Input: part model. Units: mm. Frame: model coordinates. Face numbers are marked on the shaded views. A direction names the side the tool comes from. Coordinates: 2 decimals unless noted, no trailing zeros. Order: outer loops, then holes, each group sorted by start corner. A loop starts at its lowest first (then second) coordinate and runs counter-clockwise, first axis right, second up. Notation, with made-up numbers: (82, 50.25) -> (108, 50.25) arc R35 ccw to (108, 86.25) -> close; hole circle Ø6 at (-16, 53.25). An arc over 180 degrees is marked (long way). One line per question, with ' | ' between items.
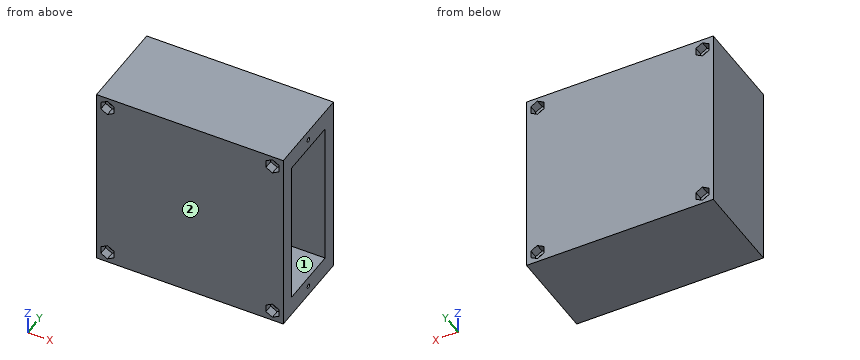
```python
from build123d import *

# Parameters (mm, degrees)
ESBO_O1_W                = 86
ESBO_O1_H                = 86
RESSALTO_EXTRUS_O1_DEPTH = 21
ESBO_O2_W                = 68
ESBO_O2_H                = 28
CORTE_EXTRUS_O1_DEPTH    = 78
ESBO_O6_R                = 1.65
CORTE_EXTRUS_O3_DEPTH    = 9
CORTE_EXTRUS_O4_DEPTH    = 4
ESPELHAR2_COPY_1_DEPTH   = 4
CORTE_EXTRUS_O5_START    = -9
ESBO_O8_R                = 1.65
CORTE_EXTRUS_O5_DEPTH    = 9
ESPELHAR4_COPY_1_DEPTH   = 4
ESPELHAR4_COPY_2_DEPTH   = 4
ESPELHAR4_COPY_3_DEPTH   = 4
ESBO_O9_R                = 1
CORTE_EXTRUS_O6_DEPTH    = 6


with BuildPart() as part:
    # Esboço1 → Ressalto-extrusão1 (new, symmetric)
    with BuildSketch(Plane(origin=(0, 0, 0), x_dir=(1, 0, 0), z_dir=(0, 1, 0))):
        Rectangle(ESBO_O1_W, ESBO_O1_H)
    extrude(amount=RESSALTO_EXTRUS_O1_DEPTH, both=True)

    # Esboço2 → Corte-extrusão1 (cut)
    with BuildSketch(Plane(origin=(43, 0, 0), x_dir=(0, 0, -1), z_dir=(1, 0, 0))):
        Rectangle(ESBO_O2_W, ESBO_O2_H)
    extrude(amount=-CORTE_EXTRUS_O1_DEPTH, mode=Mode.SUBTRACT)

    # Esboço6 → Corte-extrusão3 (cut)
    with BuildSketch(Plane(origin=(0, 21, 0), x_dir=(1, 0, 0), z_dir=(0, 1, 0))):
        with Locations(Location((-38, -38, 0), (0, 0, 270))):
            Circle(ESBO_O6_R)
        with Locations(Location((-38, 38, 0), (0, 0, 270))):
            Circle(ESBO_O6_R)
        with Locations(Location((38, 38, 0), (0, 0, 270))):
            Circle(ESBO_O6_R)
        with Locations(Location((38, -38, 0), (0, 0, 270))):
            Circle(ESBO_O6_R)
    extrude(amount=-CORTE_EXTRUS_O3_DEPTH, mode=Mode.SUBTRACT)

    # Esboço7 → Corte-extrusão4 (cut)
    with BuildSketch(Plane(origin=(0, 21, 0), x_dir=(1, 0, 0), z_dir=(0, 1, 0))):
        Polygon((-38, -34.535898385), (-41, -36.267949192), (-41, -39.732050808), (-38, -41.464101615), (-35, -39.732050808), (-35, -36.267949192), align=None)
    corte_extrus_o4 = extrude(amount=-CORTE_EXTRUS_O4_DEPTH, mode=Mode.SUBTRACT)

    # Espelhar1: Corte-extrusão4 across plane
    add(corte_extrus_o4.mirror(Plane.XY), mode=Mode.SUBTRACT)

    # Espelhar2: Corte-extrusão4 across plane
    add(corte_extrus_o4.mirror(Plane(origin=(0, 0, 0), x_dir=(0, 0, 1), z_dir=(1, 0, 0))), mode=Mode.SUBTRACT)

    # Espelhar2 copy 1 sketch → Espelhar2 copy 1 (cut)
    with BuildSketch(Plane(origin=(0, 21, 0), x_dir=(-1, 0, 0), z_dir=(0, 1, 0))):
        Polygon((-38, -34.535898385), (-41, -36.267949192), (-41, -39.732050808), (-38, -41.464101615), (-35, -39.732050808), (-35, -36.267949192), align=None)
    extrude(amount=-ESPELHAR2_COPY_1_DEPTH, mode=Mode.SUBTRACT)

    # Esboço8 → Corte-extrusão5 (cut)
    with BuildSketch(Plane.XZ.offset(21).offset(CORTE_EXTRUS_O5_START)):
        with Locations(Location((38, 38, 0), (0, 0, 90))):
            Circle(ESBO_O8_R)
        with Locations(Location((38, -38, 0), (0, 0, 90))):
            Circle(ESBO_O8_R)
        with Locations(Location((-38, -38, 0), (0, 0, 90))):
            Circle(ESBO_O8_R)
        with Locations(Location((-38, 38, 0), (0, 0, 90))):
            Circle(ESBO_O8_R)
    extrude(amount=CORTE_EXTRUS_O5_DEPTH, mode=Mode.SUBTRACT)

    # Espelhar4: Corte-extrusão4 across plane
    add(corte_extrus_o4.mirror(Plane.ZX), mode=Mode.SUBTRACT)

    # Espelhar4 copy 1 sketch → Espelhar4 copy 1 (cut)
    with BuildSketch(Plane.XZ.offset(21)):
        Polygon((-38, -34.535898385), (-41, -36.267949192), (-41, -39.732050808), (-38, -41.464101615), (-35, -39.732050808), (-35, -36.267949192), align=None)
    extrude(amount=-ESPELHAR4_COPY_1_DEPTH, mode=Mode.SUBTRACT)

    # Espelhar4 copy 2 sketch → Espelhar4 copy 2 (cut)
    with BuildSketch(Plane(origin=(0, -21, 0), x_dir=(-1, 0, 0), z_dir=(0, -1, 0))):
        Polygon((-38, -34.535898385), (-41, -36.267949192), (-41, -39.732050808), (-38, -41.464101615), (-35, -39.732050808), (-35, -36.267949192), align=None)
    extrude(amount=-ESPELHAR4_COPY_2_DEPTH, mode=Mode.SUBTRACT)

    # Espelhar4 copy 3 sketch → Espelhar4 copy 3 (cut)
    with BuildSketch(Plane(origin=(0, -21, 0), x_dir=(-1, 0, 0), z_dir=(0, -1, 0))):
        Polygon((-38, 34.535898385), (-41, 36.267949192), (-41, 39.732050808), (-38, 41.464101615), (-35, 39.732050808), (-35, 36.267949192), align=None)
    extrude(amount=-ESPELHAR4_COPY_3_DEPTH, mode=Mode.SUBTRACT)

    # Esboço9 → Corte-extrusão6 (cut)
    with BuildSketch(Plane(origin=(43, 0, 0), x_dir=(0, 0, -1), z_dir=(1, 0, 0))):
        with Locations((-38.5, 0)):
            Circle(ESBO_O9_R)
        with Locations((38.5, 0)):
            Circle(ESBO_O9_R)
    extrude(amount=-CORTE_EXTRUS_O6_DEPTH, mode=Mode.SUBTRACT)


solid = part.part
```
1. Access query for the marked faces 1 and 2. Directions: +Z, -Z, +X, -X, +Y, -Y. A direction counts if a zero-diameter tool reaches every point of the face in a straight line with its end or side. Return the directions, or none.
Recorded:
face 1: +X | face 2: +Z, -Z, +X, -X, -Y
2. Cut plane B-B, the plane x = 26. Return loops of the section in (y, z), and give its area (3 significant figures).
Recorded:
outline: (-21, -43) -> (21, -43) -> (21, 43) -> (-21, 43) -> close; hole (-14, -34) -> (14, -34) -> (14, 34) -> (-14, 34) -> close | area: 1,710 mm^2
3. Cut plane C-C, the plane y = 7. Return loops of the section in (x, z), and give its area (3 significant figures).
Recorded:
outline: (-43, -43) -> (43, -43) -> (43, -34) -> (-35, -34) -> (-35, 34) -> (43, 34) -> (43, 43) -> (-43, 43) -> close | area: 2,090 mm^2
4. Pin query (flat end, axial travel): pin 1 Ø1.5 at (y, z) = (3, -17.5) entering from +X; pin 2 Ø0.6 at (y, z) = (0, 39) entering from +X; pin 3 Ø3.5 at (x, z) = (-38.5, -38) entering from -Y. Return the tip coordinate at first contact, or that it passes through.
Recorded:
pin 1: stops at x = -35 | pin 2: stops at x = 37 | pin 3: stops at y = -17
5. Cut plane A-A, the plane z = 25. Return loops of the section in (x, y), and give its area (3 significant figures).
Recorded:
outline: (-43, -21) -> (43, -21) -> (43, -14) -> (-35, -14) -> (-35, 14) -> (43, 14) -> (43, 21) -> (-43, 21) -> close | area: 1,430 mm^2
6. Ray query, line 1 (X direction, y = 13.65, z = 38); line 2 (Y direction, x = -7, z = 25); line 3 (Z direction, x = -20.5, y = -9.5). Return the intervals inside material, ascending. Write a range as [from, to].
Recorded:
line 1: x = [-43, -39.65], [-36.35, 36.35], [39.65, 43] | line 2: y = [-21, -14], [14, 21] | line 3: z = [-43, -34], [34, 43]
